Can you work these out from the model? Positions are in its coordinate system, mm. A direction names the side the tool comes from. Coordinates: 2 decimals unless noted, no trailing zeros. Order: outer loops, then holes, each group sorted by start corner. A loop starts at its lowest first (then second) coordinate and runs counter-clockwise, first axis right, second up.
```python
from build123d import *

# Parameters (mm, degrees)
SKETCH1_R           = 87.5
BOSS_EXTRUDE1_DEPTH = 7
SKETCH2_R           = 67.5
BOSS_EXTRUDE2_DEPTH = 3
SKETCH3_R           = 2.5
CUT_EXTRUDE1_DEPTH  = 124.941518467
SKETCH4_R           = 28
BOSS_EXTRUDE3_DEPTH = 11
BOSS_EXTRUDE4_START = 11
SKETCH6_R           = 28
BOSS_EXTRUDE4_DEPTH = 11
CUT_EXTRUDE2_DEPTH  = 128.814318447


with BuildPart() as part:
    # Sketch1 → Boss-Extrude1 (new body)
    with BuildSketch(Plane(origin=(0, 0, 0), x_dir=(0, 0, -1), z_dir=(1, 0, 0))):
        Circle(SKETCH1_R)
    extrude(amount=BOSS_EXTRUDE1_DEPTH)

    # Sketch2 → Boss-Extrude2 (add)
    with BuildSketch(Plane(origin=(7, 0, 0), x_dir=(0, 0, -1), z_dir=(1, 0, 0))):
        Circle(SKETCH2_R)
    extrude(amount=BOSS_EXTRUDE2_DEPTH)

    # Sketch3 → Cut-Extrude1 (cut, through all)
    with BuildSketch(Plane(origin=(7, 0, 0), x_dir=(0, 0, -1), z_dir=(1, 0, 0))):
        with Locations((0, -80)):
            Circle(SKETCH3_R)
        with Locations((-69.282032303, -40)):
            Circle(SKETCH3_R)
        with Locations((-69.282032303, 40)):
            Circle(SKETCH3_R)
        with Locations((0, 80)):
            Circle(SKETCH3_R)
        with Locations((69.282032303, 40)):
            Circle(SKETCH3_R)
        with Locations((69.282032303, -40)):
            Circle(SKETCH3_R)
    extrude(amount=-CUT_EXTRUDE1_DEPTH, mode=Mode.SUBTRACT)

    # Sketch4 → Boss-Extrude3 (add)
    with BuildSketch(Plane(origin=(10, 0, 0), x_dir=(0, 0, -1), z_dir=(1, 0, 0))):
        Circle(SKETCH4_R)
    extrude(amount=BOSS_EXTRUDE3_DEPTH)

    # Sketch6 → Boss-Extrude4 (add)
    with BuildSketch(Plane.ZY.offset(BOSS_EXTRUDE4_START)):
        with Locations(Location((0, 0, 0), (0, 0, 180))):
            Circle(SKETCH6_R)
    extrude(amount=-BOSS_EXTRUDE4_DEPTH)

    # Sketch8 → Cut-Extrude2 (cut, through all)
    with BuildSketch(Plane(origin=(21, 0, 0), x_dir=(0, 0, -1), z_dir=(1, 0, 0))):
        with BuildLine():
            Line((-3, 16.733200531), (-3, 13.674794331))
            ThreePointArc((-3, 13.674794331), (-7, 12.124355653), (-10.342719282, 9.435473377))
            Line((-10.342719282, 9.435473377), (-12.991376746, 10.964676477))
            ThreePointArc((-12.991376746, 10.964676477), (-14.722431864, 8.5), (-15.991376746, 5.768524054))
            Line((-15.991376746, 5.768524054), (-13.342719282, 4.239320954))
            ThreePointArc((-13.342719282, 4.239320954), (-14, 0), (-13.342719282, -4.239320954))
            Line((-13.342719282, -4.239320954), (-15.991376746, -5.768524054))
            ThreePointArc((-15.991376746, -5.768524054), (-14.722431864, -8.5), (-12.991376746, -10.964676477))
            Line((-12.991376746, -10.964676477), (-10.342719282, -9.435473377))
            ThreePointArc((-10.342719282, -9.435473377), (-7, -12.124355653), (-3, -13.674794331))
            Line((-3, -13.674794331), (-3, -16.733200531))
            ThreePointArc((-3, -16.733200531), (0, -17), (3, -16.733200531))
            Line((3, -16.733200531), (3, -13.674794331))
            ThreePointArc((3, -13.674794331), (7, -12.124355653), (10.342719282, -9.435473377))
            Line((10.342719282, -9.435473377), (12.991376746, -10.964676477))
            ThreePointArc((12.991376746, -10.964676477), (14.722431864, -8.5), (15.991376746, -5.768524054))
            Line((15.991376746, -5.768524054), (13.342719282, -4.239320954))
            ThreePointArc((13.342719282, -4.239320954), (14, 0), (13.342719282, 4.239320954))
            Line((13.342719282, 4.239320954), (15.991376746, 5.768524054))
            ThreePointArc((15.991376746, 5.768524054), (14.722431864, 8.5), (12.991376746, 10.964676477))
            Line((12.991376746, 10.964676477), (10.342719282, 9.435473377))
            ThreePointArc((10.342719282, 9.435473377), (7, 12.124355653), (3, 13.674794331))
            Line((3, 13.674794331), (3, 16.733200531))
            ThreePointArc((3, 16.733200531), (0, 17), (-3, 16.733200531))
        make_face()
    extrude(amount=-CUT_EXTRUDE2_DEPTH, mode=Mode.SUBTRACT)


solid = part.part
```
1. On a 3-axis mill with a long thin cutter (end or side, diameter ignored), from which of +Z, -Z, +X, -X, +Y, -Y can I reach the whole of each face in a straight line? I mean faces 4 (the cylindrical face through (5.22, 8.54, 14.7)), 5 (the cylindrical face through (8.48, -41.07, 53.57)), 6 (the flat face through (21, 13, -6)). Say none if no direction works.
Completed:
face 4: +X, -X
face 5: +X
face 6: +Z, -Z, +X, +Y, -Y
2. Imagine slicing it at D-D on y = -40. Please give me the cut outline in (x, z).
Completed:
outline: (0, -77.82) - (7, -77.82) - (7, -71.78) - (0, -71.78) - close; (0, -66.78) - (7, -66.78) - (7, -54.37) - (10, -54.37) - (10, 54.37) - (7, 54.37) - (7, 66.78) - (0, 66.78) - close; (0, 71.78) - (7, 71.78) - (7, 77.82) - (0, 77.82) - close
3. Imagine slicing it at B-B on x = -8. Please give me the cut outline in (y, z).
Completed:
outline: circle Ø56 at (0, 0); hole (-16.73, -3) - (-13.67, -3) arc R14 ccw to (-9.44, -10.34) - (-10.96, -12.99) arc R17 ccw to (-5.77, -15.99) - (-4.24, -13.34) arc R14 ccw to (4.24, -13.34) - (5.77, -15.99) arc R17 ccw to (10.96, -12.99) - (9.44, -10.34) arc R14 ccw to (13.67, -3) - (16.73, -3) arc R17 ccw to (16.73, 3) - (13.67, 3) arc R14 ccw to (9.44, 10.34) - (10.96, 12.99) arc R17 ccw to (5.77, 15.99) - (4.24, 13.34) arc R14 ccw to (-4.24, 13.34) - (-5.77, 15.99) arc R17 ccw to (-10.96, 12.99) - (-9.44, 10.34) arc R14 ccw to (-13.67, 3) - (-16.73, 3) arc R17 ccw to start
4. Imagine slicing it at A-A on y = 0. Please give me the cut outline in (x, z).
Completed:
outline: (-11, -28) - (0, -28) - (0, -87.5) - (7, -87.5) - (7, -67.5) - (10, -67.5) - (10, -28) - (21, -28) - (21, -14) - (-11, -14) - close; (-11, 14) - (21, 14) - (21, 28) - (10, 28) - (10, 67.5) - (7, 67.5) - (7, 87.5) - (0, 87.5) - (0, 28) - (-11, 28) - close
5. I'm going to push flat-ended pins straight in: pin 1 (1.5 mm diameter, centred on x = 12.5, y = -14.5, fed in from +Z); pin 2 (6.5 mm diameter, centred on y = -40, z = 69.28, fed in from -X); pin 3 (8 mm diameter, centred on y = 80, z = 0, fed in from +X); pin 4 (3 mm diameter, centred on y = 40, z = -69.28, fed in from +X). Where does each tip first touch, or does it pass through?
Completed:
pin 1: stops at z = 24.39
pin 2: stops at x = 0
pin 3: stops at x = 7
pin 4: passes through
6. Please list where these lines run through material, in increasing order: probe 1 along Y at (x, z) = (3.5, 0); probe 2 along Y at (x, z) = (4, 69); probe 3 along X at (y, z) = (-59, -21).
Completed:
probe 1: y = -87.5 to -82.5, -77.5 to -17, 17 to 77.5, 82.5 to 87.5
probe 2: y = -53.81 to -42.48, -37.52 to 37.52, 42.48 to 53.81
probe 3: x = 0 to 10
7. Thinking about a two-plate mould opening in Z: for faces 1 (the flat face through (10, -29, 1)), 2 (the cylindrical face through (-5.577, 10.724, -25.865)), 3 (the cylindrical face through (5.224, -12.094, 7.052)), which applies, pulls with the +Z half, pulls with the -Z half, needs draft (parallel to the pull), parting line crosses it, or undercut?
Completed:
face 1: needs draft
face 2: parting line crosses it
face 3: undercut
8. Imagine slicing it at C-C on z = -32. Please give me the cut outline in (x, y).
Completed:
outline: (0, -81.44) - (7, -81.44) - (7, -59.43) - (10, -59.43) - (10, 59.43) - (7, 59.43) - (7, 81.44) - (0, 81.44) - close
